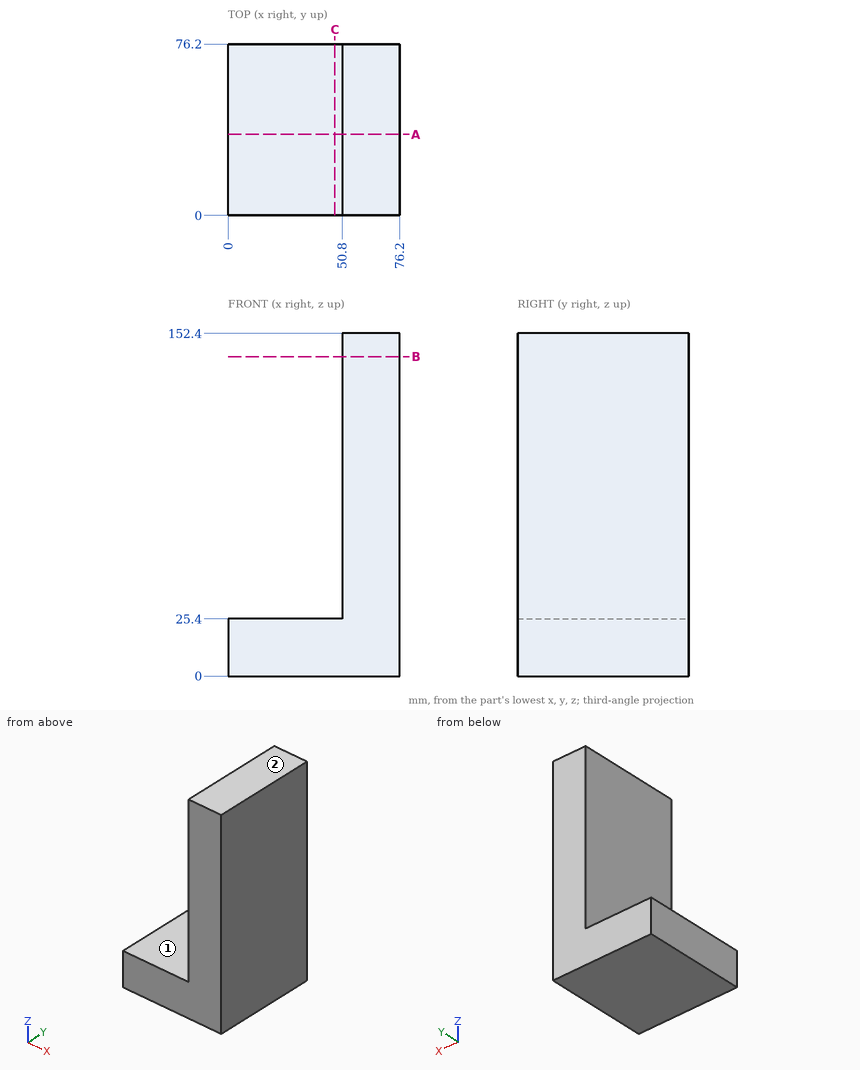
Geometry: see drawing. Coordinates: mm, zero at the bounding-box minimum. A direction names the side the tool comes from. Round coordinates to 2 decimals unless told otherwise and drop trailing zeros. Write each loop counter-clockwise with the first axis right and the second up, starting at its lowest first coordinate (ties: lowest second). Pieces come first, ordered by that corner, then holes. Notation, with made-up numbers: (-38, 42.25) -> (-24, 42.25) arc R29 cw to (-24, 72.25) -> close; hole circle Ø8 at (68.25, 66.25). An arc over 180 degrees is marked (long way). Answer as CSV lines item,"result".
1. Section A-A (y = 36). Return the cut outline in (x, z).
Geometry says:
outline,"(0, 0) -> (76.2, 0) -> (76.2, 152.4) -> (50.8, 152.4) -> (50.8, 25.4) -> (0, 25.4) -> close"
2. Section B-B (z = 142). Return the cut outline in (x, y).
Geometry says:
outline,"(50.8, 0) -> (76.2, 0) -> (76.2, 76.2) -> (50.8, 76.2) -> close"
3. Reachability of the marked faces 1 and 2 from +Z, -Z, +X, -X, +Y, -Y: full face, straight path, thin tool, end or side. Return the list, or none.
Geometry says:
face 1,"+Z, -X, +Y, -Y"
face 2,"+Z, +X, -X, +Y, -Y"
4. Ray query, L1, parallel to Z at x = 19, y = 26.5; L2, parallel to X at y = 25, z = 113. Return the intervals inside material, ascending. Write a range as [from, to].
Geometry says:
L1,"z = [0, 25.4]"
L2,"x = [50.8, 76.2]"
5. Section C-C (x = 47.5). Return the cut outline in (y, z), plus the area to 3 significant figures.
Geometry says:
outline,"(0, 0) -> (76.2, 0) -> (76.2, 25.4) -> (0, 25.4) -> close"
area,"1,940 mm^2"
6. Contact query for a flat-ended pin moving along its axis: P1, Ø1, axis at y = 66, z = 56, coming from the -X side. Output: stop coordinate, or through.
Geometry says:
P1,"stops at x = 50.8"
